```python
from build123d import *

# Parameters (mm, degrees)
BOSS_EXTRUDE2_DEPTH = 90
SKETCH2_R           = 5
CUT_EXTRUDE1_DEPTH  = 540.043745906


with BuildPart() as part:
    # Sketch1 → Boss-Extrude2 (new body)
    with BuildSketch(Plane.XY):
        with BuildLine():
            Line((20, 29.6), (510, 29.6))
            ThreePointArc((510, 29.6), (517.071067812, 26.671067812), (520, 19.6))
            Line((520, 19.6), (520, 0))
            Line((520, 0), (530, 0))
            Line((530, 0), (530, 19.6))
            ThreePointArc((530, 19.6), (524.142135624, 33.742135624), (510, 39.6))
            Line((510, 39.6), (20, 39.6))
            ThreePointArc((20, 39.6), (5.857864376, 33.742135624), (0, 19.6))
            Line((0, 19.6), (0, 0))
            Line((0, 0), (10, 0))
            Line((10, 0), (10, 19.6))
            ThreePointArc((10, 19.6), (12.928932188, 26.671067812), (20, 29.6))
        make_face()
    extrude(amount=BOSS_EXTRUDE2_DEPTH)

    # Sketch2 → Cut-Extrude1 (cut, through all)
    with BuildSketch(Plane.ZY):
        with Locations((20, 10)):
            Circle(SKETCH2_R)
        with Locations(Location((70, 10, 0), (0, 0, 180))):
            Circle(SKETCH2_R)
    extrude(amount=-CUT_EXTRUDE1_DEPTH, mode=Mode.SUBTRACT)


solid = part.part
```
Geometry check sheet. Reference: the model listing, model coordinates, mm. A direction names the side the tool comes from. Give positions to 0.01 mm unless a question says otherwise; leave off trailing zeros. Loops run counter-clockwise (first coordinate to the right, second up) from the corner with the lowest first, then second, coordinate; pieces in that order, holes last. Notation, with made-up numbers: M 44,74.5 L 80,74.5 A30 ccw 80,107.5 Z; hole C -4.5,85.5 d8. An arc over 180 degrees is marked long. Answer as CSV lines item,"result".
Item 1: Cross-section at A-A on y = 10. Record the cut outline in (x, z).
Values:
outline,"M 0,0 L 10,0 L 10,15 L 0,15 Z; M 0,25 L 10,25 L 10,65 L 0,65 Z; M 0,75 L 10,75 L 10,90 L 0,90 Z; M 520,0 L 530,0 L 530,15 L 520,15 Z; M 520,25 L 530,25 L 530,65 L 520,65 Z; M 520,75 L 530,75 L 530,90 L 520,90 Z"
Item 2: Cross-section at D-D on x = 424. Record the cut outline in (y, z), and give its area (3 significant figures).
Values:
outline,"M 29.6,0 L 39.6,0 L 39.6,90 L 29.6,90 Z"
area,"900 mm²"
Item 3: Cross-section at B-B on z = 20. Record the cut outline in (x, y).
Values:
outline,"M 0,0 L 10,0 L 10,5 L 0,5 Z; M 0,15 L 10,15 L 10,19.6 A10 cw 20,29.6 L 510,29.6 A10 cw 520,19.6 L 520,15 L 530,15 L 530,19.6 A20 ccw 510,39.6 L 20,39.6 A20 ccw 0,19.6 Z; M 520,0 L 530,0 L 530,5 L 520,5 Z"
Item 4: Access from +Z, -Z, +X, -X, +Y, -Y to the whole of each face (thin tool, end or side, straight path). Record for faces 1 (the flat face through (5, 0, 44)), 2 (the cylindrical face through (12.85, 26.59, 44.37)).
Values:
face 1,"+Z, -Z, +X, -X, -Y"
face 2,"+Z, -Z, -Y"
Item 5: Cross-section at C-C on z = 48.5. Record the cut outline in (x, y).
Values:
outline,"M 0,0 L 10,0 L 10,19.6 A10 cw 20,29.6 L 510,29.6 A10 cw 520,19.6 L 520,0 L 530,0 L 530,19.6 A20 ccw 510,39.6 L 20,39.6 A20 ccw 0,19.6 Z"
Item 6: Depth check by flat-ended pin: P1, Ø2, axis at y = 26, z = 55.5, coming from the +X side; P2, Ø5, axis at y = 32.5, z = 67.5, coming from the +X side; P3, Ø12, axis at x = 94, z = 68.5, coming from the -Y side. Enter the tip coordinate at first touch or a pass-through.
Values:
P1,"stops at x = 529.26"
P2,"stops at x = 527.08"
P3,"stops at y = 29.6"
Item 7: Release check for a two-part mould opening along Y. For faces 3 (the flat face through (10, 10, 44)), 4 (the cylindrical face through (524.297, 33.586, 44.37)), 5 (the cylindrical face through (516.99, 26.75, 44.37)), 6 (the cylindrical face through (524.93, 11.915, 65.381)) record: pulls with the +Y half, pulls with the -Y half, needs draft (parallel to the pull), parting line crosses it, or undercut.
Values:
face 3,"needs draft"
face 4,"pulls with the +Y half"
face 5,"pulls with the -Y half"
face 6,"undercut"
Item 8: Material ranges on line 1 (X direction, y = 15, z = 57); line 2 (Y direction, x = 81, z = 44.5); line 3 (X direction, y = 24.5, z = 45), recorded low to high.
Values:
line 1,"x = 0 to 10, 520 to 530"
line 2,"y = 29.6 to 39.6"
line 3,"x = 0.61 to 11.28, 518.72 to 529.39"
